Could you check a few things on this drawing? It's one solid part, dimensions in mm from its lowest x, y, z. A direction names the side the tool comes from. Round coordinates to 2 decimals unless told otherwise and drop trailing zeros. Order: outer loops, then holes, each group sorted by start corner. A loop starts at its lowest first (then second) coordinate and runs counter-clockwise, first axis right, second up. Notation, with made-up numbers: (-27, 52) -> (-21, 52) arc R36 ccw to (-21, 87) -> close; hole circle Ø1 at (1, 15). An arc over 180 degrees is marked (long way). Use a Markdown table: item, result. Add a question column.
(1) If I drill on probe 1 along Y at (x, z) = (26, 2.3); probe 2 along Y at (x, z) = (4, 1.4); probe 3 along X at (y, z) = (10, 0.9), over which ranges is the centre line in solid material (lowest first)?
(2) I want a section at B-B, the plane y = 26. Please give me the cut outline in (x, z), then the cut area to 3 significant figures.
(3) I want a section at A-A, the plane z = 2.2. Give the number of separate pieces and of enclosed holes in the cut face, then the cut area to 3 significant figures.
(4) Thinking about a two-plate mould opening in X: for the marked faces 1, 2 and 3, which applies, pulls with the +X half, pulls with the -X half, needs draft (parallel to the pull), parting line crosses it, or undercut?
(5) I want a section at C-C, the plane x = 36.5. Please give me the cut outline in (y, z), then the cut area to 3 significant figures.
(6) On a 3-axis mill with a long thin cutter (end or side, diameter ignored), from which of +Z, -Z, +X, -X, +Y, -Y can I reach the whole of each face in a straight line? I mean the marked faces 4, 5 and 6. Say none if no direction works.
(7) I'm going to push flat-ended pins straight in: P1, Ø5, axis at x = 16.5, y = 26, coming from the -Z side; P2, Ø0.9, axis at y = 6.5, z = 2, coming from the -X side; P3, Ø1.5, axis at y = 10, z = 1.5, coming from the +X side; P4, Ø0.9, axis at x = 42, z = 1.5, coming from the +Y side. Where does each tip first touch, or does it pass through?
(8) I want a section at D-D, the plane x = 17.5. Please give me the cut outline in (y, z), then the cut area to 3 significant figures.
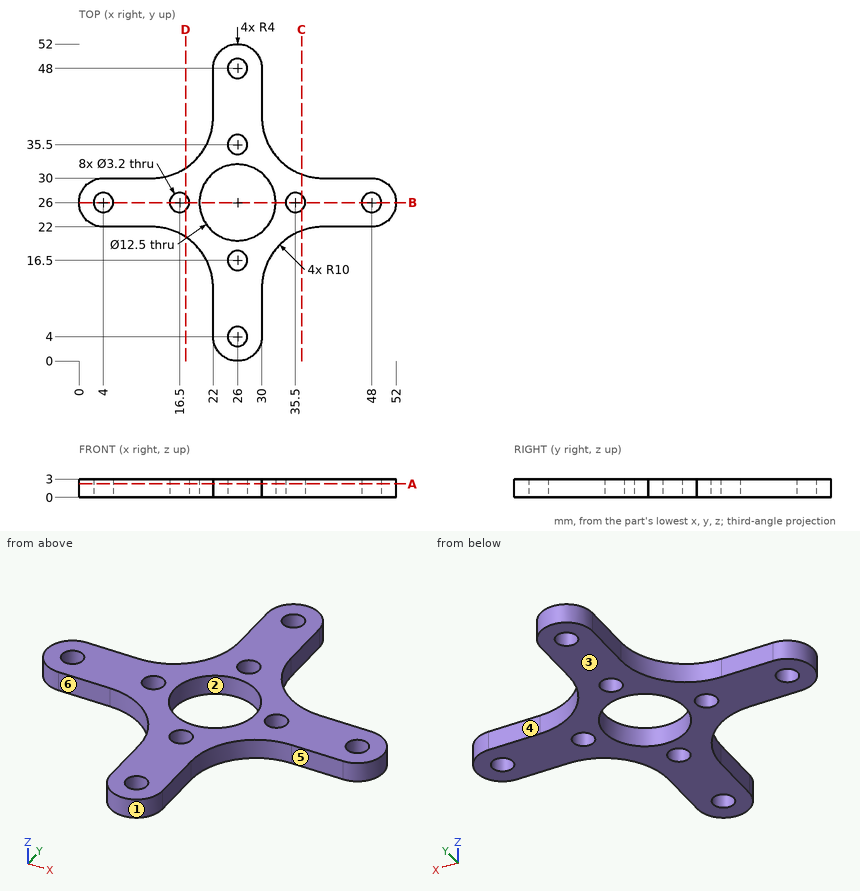
Taken from the geometry:
| question | item | result |
|---|---|---|
| 1 | probe 1 | y = 0 to 2.4, 5.6 to 14.9, 18.1 to 19.75, 32.25 to 33.9, 37.1 to 46.4, 49.6 to 52 |
| 1 | probe 2 | y = 22 to 24.4, 27.6 to 30 |
| 1 | probe 3 | x = 22 to 30 |
| 2 | outline | (0, 0) -> (2.4, 0) -> (2.4, 3) -> (0, 3) -> close; (5.6, 0) -> (14.9, 0) -> (14.9, 3) -> (5.6, 3) -> close; (18.1, 0) -> (19.75, 0) -> (19.75, 3) -> (18.1, 3) -> close; (32.25, 0) -> (33.9, 0) -> (33.9, 3) -> (32.25, 3) -> close; (37.1, 0) -> (46.4, 0) -> (46.4, 3) -> (37.1, 3) -> close; (49.6, 0) -> (52, 0) -> (52, 3) -> (49.6, 3) -> close |
| 2 | area | 80.1 mm2 |
| 3 | separate pieces | 1 |
| 3 | enclosed holes | 9 |
| 3 | area | 639 mm2 |
| 4 | face 1 | parting line crosses it |
| 4 | face 2 | undercut |
| 4 | face 3 | needs draft |
| 5 | outline | (21.37, 0) -> (24.75, 0) -> (24.75, 3) -> (21.37, 3) -> close; (27.25, 0) -> (30.63, 0) -> (30.63, 3) -> (27.25, 3) -> close |
| 5 | area | 20.3 mm2 |
| 6 | face 4 | +Z, -Z, +X, +Y |
| 6 | face 5 | +Z, -Z, +X, -Y |
| 6 | face 6 | +Z, -Z, -X, -Y |
| 7 | P1 | stops at z = 0 |
| 7 | P2 | stops at x = 22 |
| 7 | P3 | stops at x = 30 |
| 7 | P4 | stops at y = 30 |
| 8 | outline | (20.35, 0) -> (24.75, 0) -> (24.75, 3) -> (20.35, 3) -> close; (27.25, 0) -> (31.65, 0) -> (31.65, 3) -> (27.25, 3) -> close |
| 8 | area | 26.4 mm2 |
